Autodesk Inventor part; units mm, degrees
ref_plane "YZ Plane" through (0, 0, 0) normal (1, 0, 0) x (0, 1, 0)
ref_plane "XZ Plane" through (0, 0, 0) normal (0, 1, 0) x (-1, 0, 0)
ref_plane "XY Plane" through (0, 0, 0) normal (0, 0, 1) x (1, 0, 0)
sketch "Sketch1" plane through (0, 0, 0) normal (0, 0, 1) x (1, 0, 0)
  line L0 (0, 46.5) -> (46.5, 46.5)
  line L1 (46.5, 46.5) -> (46.5, 0)
  line L2 (46.5, 0) -> (46.5, -46.5)
  line L3 (46.5, -46.5) -> (0, -46.5)
  line L4 (0, -46.5) -> (-46.5, -46.5)
  line L5 (-46.5, -46.5) -> (-46.5, 0)
  line L6 (-46.5, 0) -> (-46.5, 46.5)
  line L7 (-46.5, 46.5) -> (0, 46.5)
  point P0 (0, 0)
  dimension "d82" = 46.5
  dimension "d83" = 46.5
  dimension "d84" = 93
  dimension "d85" = 93
extrude "Plate" add sketch "Sketch1" along normal blind 1
sketch "Sketch2" plane through (0, 0, 1) normal (0, 0, 1) x (1, 0, 0)
  circle A0 centre (-23.5, -28.5) radius 8.25
  circle A1 centre (-12.4, -28.5) radius 1.7
  circle A2 centre (-34.6, -28.5) radius 1.7
  line L0 (-46.5, 46.5) -> (-46.5, -46.5)
  line L1 (-46.5, -46.5) -> (46.5, -46.5)
  point P0 (0, 0)
  dimension "d6" = 16.5
  dimension "d8" = 3.4
  dimension "d29" = 11.1
  dimension "d30" = 11.1
  dimension "d93" = 23
  dimension "d94" = 18
extrude "DIN hole" cut sketch "Sketch2" against normal through all
pattern_linear "Rectangular Pattern1" count 2 spacing 25 along (0, 1, 0) of "DIN hole"
sketch "Sketch4" plane through (0, 0, 1) normal (0, 0, 1) x (1, 0, 0)
  circle A0 centre (-23.5, -28.5) radius 8.25
  point P0 (0, 0)
sketch "Sketch5" plane through (0, 0, 1) normal (0, 0, 1) x (1, 0, 0)
  line L0 (46.5, 46.5) -> (-46.5, 46.5)
  line L1 (-46.5, 46.5) -> (-46.5, -46.5)
  circle A0 centre (-32.5, 21.5) radius 4.5
  point P0 (0, 0)
  dimension "d90" = 9
  dimension "d91" = 14
  dimension "d92" = 25
extrude "LED" cut sketch "Sketch5" along normal through all both and the other way through all
pattern_linear "Rectangular Pattern3" count 2 spacing 20 along (1, 0, 0) of "LED"
sketch "Sketch6" plane through (0, 0, 1) normal (0, 0, 1) x (1, 0, 0)
  circle A0 centre (32.5, 21.5) radius 4.85
  point P0 (-26.5, 37.5)
  point P1 (0, 0)
  dimension "d61" = 9.7
extrude "BNCs" cut sketch "Sketch6" along normal through all both and the other way through all
sketch "Sketch7" plane through (0, 0, 1) normal (0, 0, 1) x (1, 0, 0)
  circle A0 centre (32.5, 21.5) radius 4.85
  circle A1 centre (10.5, 21.5) radius 4.75
  circle A2 centre (10.5, 12) radius 0.8
  point P0 (0, 0)
  dimension "d70" = 9.5
  dimension "d71" = 1.6
  dimension "d72" = 9.5
  dimension "d73" = 22
extrude "Extrusion9" cut sketch "Sketch7" against normal blind 1 contours A1 | A2
sketch "Sketch8" plane through (0, 0, 1) normal (0, 0, 1) x (1, 0, 0)
  arc A0 (36.5, 4.7427) -> (36.5, -0.7427) centre (32.5, 2) ccw
  line L0 (36.5, 2) -> (36.5, -0.7427)
  line L1 (36.5, 2) -> (36.5, 4.7427)
  point P0 (0, 0)
extrude "Extrusion10" cut sketch "Sketch8" against normal blind 10
properties part number "AmplifierPowerSupplyNew"
Check sheet for the modelled part. Datum: model origin and axes. Units: mm. Round coordinates to 2 decimals unless told otherwise and drop trailing zeros. Loops run counter-clockwise (first coordinate to the right, second up) from the corner with the lowest first, then second, coordinate; pieces in that order, holes last. Notation, with made-up numbers: (9.5, 66.25) -> (16.5, 66.25) arc R17 ccw to (16.5, 73.25) -> close; hole circle Ø9 at (56, 63.25). An arc over 180 degrees is marked (long way). Answer in a Markdown table with one row per item.
Q1. Release check for a two-part mould opening along X. For faces 1 (the face through (27.653, 2.172, 0.507)), 2 (the face through (9.88, 26.21, 0.51)), 3 (the face through (-1, 1, 0)) record: released by +X, released by -X, zero draft, split by the parting line, or undercut.
Data:
| item | result |
|---|---|
| face 1 | undercut |
| face 2 | undercut |
| face 3 | zero draft |
Q2. Go/stop test with a flat-tipped pin: P1, Ø7, axis at x = -12.5, y = 21.5, coming from the -Z side. Record where the tip stops, or that it passes through.
Data:
| item | result |
|---|---|
| P1 | passes through |
Q3. Sectioned sample at B-B on x = -34.6. Enter the section's corners in (y, z).
Data:
| item | result |
|---|---|
| outline | (-46.5, 0) -> (-30.2, 0) -> (-30.2, 1) -> (-46.5, 1) -> close; (-26.8, 0) -> (-5.2, 0) -> (-5.2, 1) -> (-26.8, 1) -> close; (-1.8, 0) -> (17.52, 0) -> (17.52, 1) -> (-1.8, 1) -> close; (25.48, 0) -> (46.5, 0) -> (46.5, 1) -> (25.48, 1) -> close |
Q4. Sectioned sample at C-C on y = -8. Enter the section's corners in (x, z).
Data:
| item | result |
|---|---|
| outline | (-46.5, 0) -> (-30.41, 0) -> (-30.41, 1) -> (-46.5, 1) -> close; (-16.59, 0) -> (46.5, 0) -> (46.5, 1) -> (-16.59, 1) -> close |
Q5. Sectioned sample at A-A on y = -28.5. Enter the section's corners in (x, z).
Data:
| item | result |
|---|---|
| outline | (-46.5, 0) -> (-36.3, 0) -> (-36.3, 1) -> (-46.5, 1) -> close; (-32.9, 0) -> (-31.75, 0) -> (-31.75, 1) -> (-32.9, 1) -> close; (-15.25, 0) -> (-14.1, 0) -> (-14.1, 1) -> (-15.25, 1) -> close; (-10.7, 0) -> (46.5, 0) -> (46.5, 1) -> (-10.7, 1) -> close |
Q6. Sectioned sample at D-D on y = 2. Enter the section's corners in (x, z), then the cut area to 3 significant figures.
Data:
| item | result |
|---|---|
| outline | (-46.5, 0) -> (-29.65, 0) -> (-29.65, 1) -> (-46.5, 1) -> close; (-17.35, 0) -> (27.65, 0) -> (27.65, 1) -> (-17.35, 1) -> close; (36.5, 0) -> (46.5, 0) -> (46.5, 1) -> (36.5, 1) -> close |
| area | 71.9 mm^2 |
Q7. Thickness scan on L1, parallel to Y at x = -23.5, z = 0.6; L2, parallel to Y at x = -12.4, z = 0.35; L3, parallel to X at y = 2, z = 0.5. Record the ranges inside material, lowest first.
Data:
| item | result |
|---|---|
| L1 | y = -46.5 to -36.75, -20.25 to -11.75, 4.75 to 46.5 |
| L2 | y = -46.5 to -30.2, -26.8 to -5.2, -1.8 to 17, 26 to 46.5 |
| L3 | x = -46.5 to -29.65, -17.35 to 27.65, 36.5 to 46.5 |
